from build123d import *

# Parameters (mm, degrees)
F0_W     = 40
F0_H     = 28
F0_W_2   = 20
F0_H_2   = 20
F1_DEPTH = 25
F2_W     = 20
F2_H     = 20
F3_DEPTH = 15
F4_W     = 40
F4_H     = 28
F5_DEPTH = 15


with BuildPart() as f1:
    # F0 (on Top) → F1 (new body)
    with BuildSketch(Plane.XY):
        Polygon((-1.226237, 20.598543), (-41.226237, 20.598543), (-41.226237, 0.598543), (-21.226237, 0.598543), (-21.226237, -19.401457), (38.773763, -19.401457), (38.773763, -7.401457), (-1.226237, -7.401457), align=None)
        with Locations((18.773763, 6.598543)):
            Rectangle(F0_W, F0_H)
        with Locations((-31.226237, -9.401457)):
            Rectangle(F0_W_2, F0_H_2)
    extrude(amount=F1_DEPTH)

    # F2 (on face) → F3 (cut)
    with BuildSketch(Plane.XY.offset(25)):
        with Locations((-31.226237, -9.401457)):
            Rectangle(F2_W, F2_H)
    extrude(amount=-F3_DEPTH, mode=Mode.SUBTRACT)

    # F4 (on face) → F5 (join)
    with BuildSketch(Plane.XY.offset(25)):
        with Locations((18.773763, 6.598543)):
            Rectangle(F4_W, F4_H)
    extrude(amount=F5_DEPTH)


solid = f1.part
For this review, take the finished solid that the model builds, in its own axes (mm). A direction names the side the tool comes from. Round coordinates to 2 decimals unless told otherwise and drop trailing zeros. Loops run counter-clockwise (first coordinate to the right, second up) from the corner with the lowest first, then second, coordinate; pieces in that order, holes last. Notation, with made-up numbers: (-32.5, -16) - (2.5, -16) arc R11 ccw to (2.5, 5) - close; hole circle Ø7 at (-28.5, -26.5). An arc over 180 degrees is marked (long way). Use one line per item in the form item = value.
Item 1: For line 1 (Y direction, x = -1, z = 26); line 2 (X direction, y = -1, z = 19); line 3 (Z direction, x = 9, y = -14.5), list the stretches that pass through material, from the lowest coordinate up.
Answers:
line_1 = -7.4 to 20.6
line_2 = -21.23 to 38.77
line_3 = 0 to 25
Item 2: Consider section D-D on x = -7. Write out the cut boundary in (y, z), then the cut area to 3 significant figures.
Answers:
outline = (-19.4, 0) - (20.6, 0) - (20.6, 25) - (-19.4, 25) - close
area = 1,000 mm^2
Item 3: Consider section B-B on z = 11. Write out the cut boundary in (x, y).
Answers:
outline = (-41.23, 0.6) - (-21.23, 0.6) - (-21.23, -19.4) - (38.77, -19.4) - (38.77, 20.6) - (-41.23, 20.6) - close
Item 4: Tool access review of faces 1 (the flat face through (-41.226, 5, 10)), 2 (the flat face through (-1.226, 6, 32)), 3 (the flat face through (-2, 20.599, 15)), 4 (the flat face through (18, -7.401, 32)), 5 (the flat face through (-21.226, -10, 18)): name each direction out of +Z, -Z, +X, -X, +Y, -Y from which nothing blocks a thin tool from reaching the whole face with its end or side.
Answers:
face_1 = +Z, -Z, -X, +Y, -Y
face_2 = +Z, -X, +Y, -Y
face_3 = +Z, -Z, +X, -X, +Y
face_4 = +Z, +X, -X, -Y
face_5 = +Z, -X, -Y
Item 5: Clearance check with flat-ended pins moving along their axes: P1, Ø16.5, axis at x = -28, z = 15, coming from the -Y side; P2, Ø4, axis at y = -1, z = 30, coming from the -X side; P3, Ø10, axis at x = 26.5, y = -13, coming from the +Z side; P4, Ø7.5, axis at y = -11, z = 19.5, coming from the -X side. State where each tip first meets the part, or that it passes through.
Answers:
P1 = -19.4
P2 = -1.23
P3 = 25
P4 = -21.23
Item 6: Consider section C-C on x = 3. Write out the cut boundary in (y, z).
Answers:
outline = (-19.4, 0) - (20.6, 0) - (20.6, 40) - (-7.4, 40) - (-7.4, 25) - (-19.4, 25) - close
Item 7: Consider section A-A on y = -5. Write out the cut boundary in (x, z), then the cut area to 3 significant figures.
Answers:
outline = (-41.23, 0) - (38.77, 0) - (38.77, 40) - (-1.23, 40) - (-1.23, 25) - (-21.23, 25) - (-21.23, 10) - (-41.23, 10) - close
area = 2,300 mm^2
